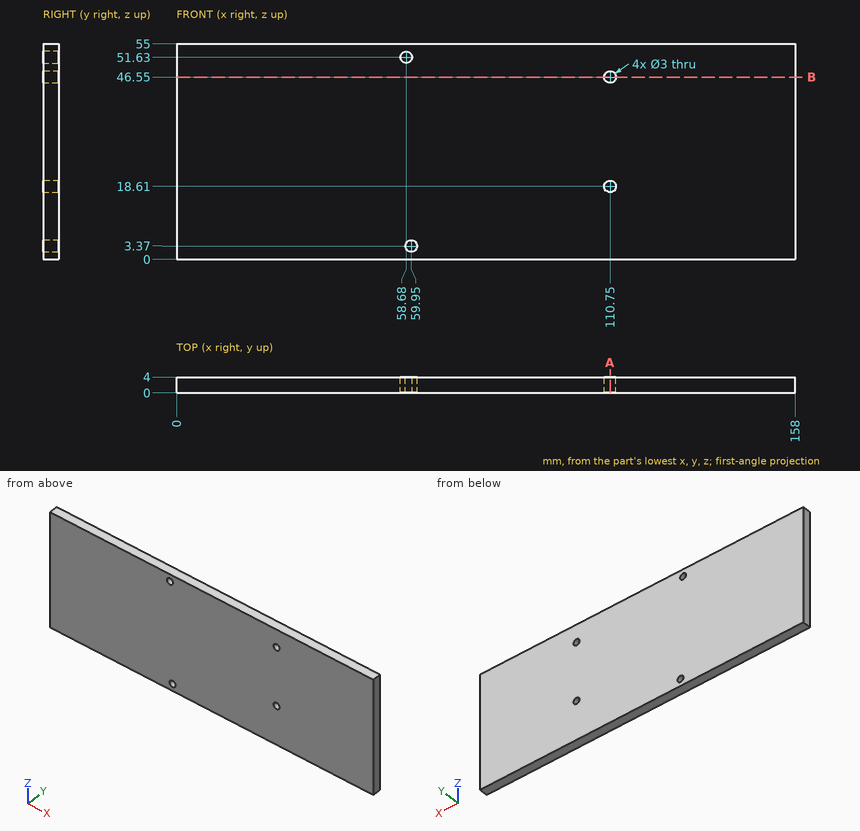
Design review of the part shown in the three views and the two pictorial views. Dimensions are in mm from the part's minimum x, y and z. Give positions to 0.01 mm unless a question says otherwise; leave off trailing zeros. Write each loop counter-clockwise with the first axis right and the second up, starting at its lowest first coordinate (ties: lowest second). Pieces come first, ordered by that corner, then holes. Notation, with made-up numbers: M 31.25,22.5 L 36.25,22.5 A29 ccw 36.25,48.5 Z; hole C -35.75,28 d9. An arc over 180 degrees is marked long. One line per item, written item: value.
1) Take a section at B-B, the plane z = 46.55. Write out the cut boundary in (x, y), then the cut area to 3 significant figures.
Results are:
outline: M 0,0 L 109.25,0 L 109.25,4 L 0,4 Z; M 112.25,0 L 158,0 L 158,4 L 112.25,4 Z
area: 620 mm²
2) Take a section at A-A, the plane x = 110.75. Write out the cut boundary in (y, z).
Results are:
outline: M 0,0 L 4,0 L 4,17.11 L 0,17.11 Z; M 0,20.11 L 4,20.11 L 4,45.05 L 0,45.05 Z; M 0,48.05 L 4,48.05 L 4,55 L 0,55 Z
3) For line 1 (Z direction, x = 110.75, y = 0.9); line 2 (X direction, y = 1.2, z = 3.37); line 3 (X direction, y = 1.5, z = 46.55), list the stretches that pass through material, from the lowest coordinate up. Write a range as from..to.
Results are:
line 1: z = 0..17.11, 20.11..45.05, 48.05..55
line 2: x = 0..58.45, 61.45..158
line 3: x = 0..109.25, 112.25..158
